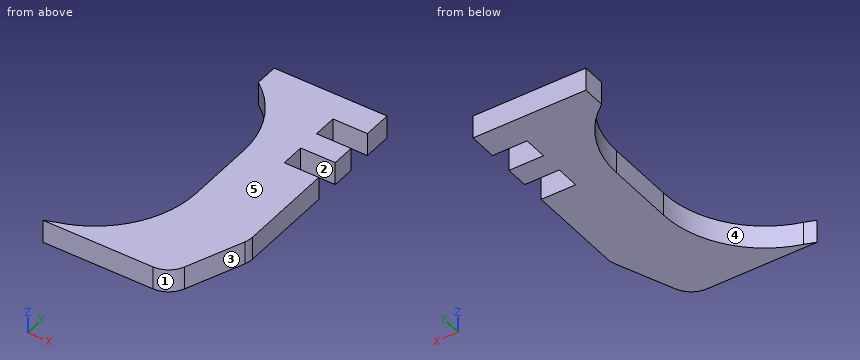
Autodesk Inventor part; units mm, degrees
ref_plane "YZ Plane" through (0, 0, 0) normal (1, 0, 0) x (0, 1, 0)
ref_plane "XZ Plane" through (0, 0, 0) normal (0, 1, 0) x (-1, 0, 0)
ref_plane "XY Plane" through (0, 0, 0) normal (0, 0, 1) x (1, 0, 0)
sketch "Sketch1" plane through (0, 0, 0) normal (0, 0, 1) x (1, 0, 0)
  arc A0 (6.0987, 0.8622) -> (22, 22) centre (0, 22) ccw
  line L0 (22, 22) -> (22, 37)
  arc A1 (22, 37) -> (13, 54.7482) centre (0, 37) ccw
  line L1 (13, 54.7482) -> (13, 66.7482)
  line L2 (22.5, 90) -> (22.5, 66.7482)
  line L3 (22.5, 90) -> (37.5, 90)
  line L4 (13, 66.7482) -> (22.5, 66.7482)
  line L5 (32.3216, 3.1515) -> (37.1457, 15.2755)
  arc A2 (37.1457, 15.2755) -> (37.5, 17.1241) centre (32.5, 17.1241) ccw
  arc A3 (27.6759, 0) -> (32.3216, 3.1515) centre (27.6759, 5) ccw
  line L6 (37.5, 53.562) -> (30, 53.562)
  line L7 (30, 53.562) -> (30, 48.362)
  line L8 (30, 48.362) -> (37.5, 48.362)
  line L9 (37.5, 43.362) -> (30, 43.362)
  line L10 (30, 43.362) -> (30, 38.162)
  line L11 (30, 38.162) -> (37.5, 38.162)
  line L12 (37.5, 90) -> (37.5, 53.562)
  line L13 (37.5, 48.362) -> (37.5, 43.362)
  line L14 (37.5, 38.162) -> (37.5, 17.1241)
  line L15 (6.0987, 0.8622) -> (3.793, 0)
  line L16 (3.793, 0) -> (27.6759, 0)
  point P0 (0, 0)
  dimension "d0" = 22
  dimension "d1" = 90
  dimension "d2" = 0
  dimension "d3" = 15
  dimension "d4" = 0
  dimension "d5" = 13
  dimension "d6" = 22
  dimension "d7" = 12
  dimension "d8" = 22.5
  dimension "d10" = 90
  dimension "d11" = 37
  dimension "d12" = 5
  dimension "d13" = 12.1241
  dimension "d14" = 5.2
  dimension "d15" = 5.2
  dimension "d16" = 5
sketch "Sketch2" plane through (0, 0, 0) normal (0, 0, 1) x (1, 0, 0)
  point P0 (0, 0)
extrude "Extrusion1" add sketch "Sketch1" along normal blind 5
sketch "Sketch3" plane through (0, 0, 5) normal (0, 0, 1) x (1, 0, 0)
  line L0 (22.5, 90) -> (22.5, 66.7482)
  line L1 (37.5, 90) -> (22.5, 90)
  point P0 (0, 0)
  point P1 (30, 86.5)
  point P2 (30, 63.5)
  dimension "d20" = 23
  dimension "d21" = 7.5
  dimension "d22" = 7.5
  dimension "d23" = 3.5
hole "Hole1" at (30, 86.5, 5) at (30, 63.5, 5) direction (0, 0, -1) diameter 3.4 end through all
sketch "Sketch4" plane through (22.5, 66.7482, 0) normal (-1, 0, 0) x (0, 0, 1)
  point P0 (0, -66.7482)
sketch "Sketch5" plane through (13, 54.7482, 0) normal (-1, 0, 0) x (0, 0, 1)
  line L0 (-13.1984, 36.8887) -> (18.4276, 36.8887)
  line L1 (18.4276, 36.8887) -> (18.4276, 5)
  line L2 (18.4276, 5) -> (-13.1984, 5)
  line L3 (-13.1984, 5) -> (-13.1984, 36.8887)
  line L4 (0, 12) -> (5, 12)
  point P0 (0, -54.7482)
  dimension "d31" = 7
extrude "Extrusion2" cut sketch "Sketch5" against normal blind 40
properties part number "CenterFinger"
Read the model definition and answer for the solid it produces. Units are mm, in the model's axes. Face numbers are marked on the shaded views. A direction names the side the tool comes from. Give positions to 0.01 mm unless a question says otherwise; leave off trailing zeros. Loops run counter-clockwise (first coordinate to the right, second up) from the corner with the lowest first, then second, coordinate; pieces in that order, holes last.
Item 1: The part is cut by section B-B (z = 0.65). Write down the section's boundary in (x, y), and give its area (3 significant figures).
Item 2: The part is cut by section C-C (y = 33). Write down the section's boundary in (x, z).
Item 3: The part is cut by section A-A (x = 34). Write down the section's boundary in (y, z).
Item 4: Find the intervals of material crossed by line 1 along Y through (x, z) = (31.5, 3.4); line 2 along Y through (x, z) = (20, 4.5); line 3 along Y through (x, z) = (18.5, 2.2), in increasing order.
Item 5: The part is cut by section D-D (x = 14.5). Write down the section's boundary in (y, z).
Item 6: For the marked faces 1 and 2, determine the directions among +Z, -Z, +X, -X, +Y, -Y from which every point of the face is accessible in a straight line to the end or side of a thin tool.
Item 7: The mould has two halves that part along Y. Classify the marked faces 3, 4 and 5: released by +Y, released by -Y, zero draft, split by the parting line, or undercut.
Item 8: Each of these flat-tipped pins is pushed along its axis until it touches: pin 1 Ø4 at (x, y) = (21, 22) entering from -Z; pin 2 Ø2.5 at (y, z) = (33, 2.5) entering from -X; pin 3 Ø2.5 at (y, z) = (52, 2.5) entering from +X. Where does it stop, or does it pass through?
Taken from the geometry:
1. outline: (3.79, 0) - (27.68, 0) arc R5 ccw to (32.32, 3.15) - (37.15, 15.28) arc R5 ccw to (37.5, 17.12) - (37.5, 38.16) - (30, 38.16) - (30, 43.36) - (37.5, 43.36) - (37.5, 48.36) - (30, 48.36) - (30, 53.56) - (37.5, 53.56) - (37.5, 59.75) - (13, 59.75) - (13, 54.75) arc R22 cw to (22, 37) - (22, 22) arc R22 cw to (6.1, 0.86) - close
1. area: 990 mm2
2. outline: (22, 0) - (37.5, 0) - (37.5, 5) - (22, 5) - close
3. outline: (7.37, 0) - (38.16, 0) - (38.16, 5) - (7.37, 5) - close; (43.36, 0) - (48.36, 0) - (48.36, 5) - (43.36, 5) - close; (53.56, 0) - (59.75, 0) - (59.75, 5) - (53.56, 5) - close
4. line 1: y = 1.78 to 38.16, 43.36 to 48.36, 53.56 to 59.75
4. line 2: y = 0 to 12.83, 46.17 to 59.75
4. line 3: y = 0 to 10.09, 48.91 to 59.75
5. outline: (0, 0) - (5.45, 0) - (5.45, 5) - (0, 5) - close; (53.55, 0) - (59.75, 0) - (59.75, 5) - (53.55, 5) - close
6. face 1: +Z, -Z, +X, -Y
6. face 2: +Z, -Z, +X
7. face 3: released by -Y
7. face 4: undercut
7. face 5: zero draft
8. pin 1: stops at z = 0
8. pin 2: stops at x = 22
8. pin 3: stops at x = 30
